Build history of the part. All positions in model axes, mm. A direction names the side the tool comes from. Coordinates: 2 decimals unless noted, no trailing zeros. Write each loop counter-clockwise with the first axis right and the second up, starting at its lowest first coordinate (ties: lowest second). Pieces come first, ordered by that corner, then holes.
```python
from build123d import *

# Parameters (mm, degrees)
SKETCH3_R   = 21.43125
SKETCH3_R_2 = 12.1539


with BuildPart() as part:
    # Sketch1 → Revolve1 (revolve)
    with BuildSketch(Plane.XY):
        Polygon((-11.786586159, -42.094950568), (8.688397797, -21.619966611), (5.298351111, -18.229919926), (-15.041929003, -38.839607724), align=None)
    revolve(axis=Axis((-26.940768363, -26.940768363, 0), (0.707106781, 0.707106781, 0)))



with BuildPart() as body_2:
    # Sketch2 → Revolve2 (revolve)
    with BuildSketch(Plane.XY):
        Polygon((16.8275, 38.1), (16.637, 9.144), (21.43125, 9.144), (21.43125, 38.1), align=None)
    revolve(axis=Axis((0, 0, 0), (0, 1, 0)))


with BuildPart() as part_1:
    add(part.part)

    add(body_2.part)  # Sweep1 merges body 2
    # Sweep1: sweep along a path in Sketch4
    with BuildLine(Plane.XY) as sweep1_path:
        ThreePointArc((-6.465784407, -6.465784407), (-1.680402618, 0.696045555), (0, 9.144))
    # Sketch3 → Sweep1 (sweep)
    with BuildSketch(Plane(origin=(-6.465784407, -6.465784407, 0), x_dir=(0, 0, -1), z_dir=(0.707106781, 0.707106781, 0))):
        Circle(SKETCH3_R)
        Circle(SKETCH3_R_2, mode=Mode.SUBTRACT)
    sweep(path=sweep1_path.line)


solid = part_1.part
```
1. Saw through at A-A on y = 31. List the corners of the cut face in (x, z), plus the area to 3 significant figures.
Computed values:
outline: circle Ø42.86 at (0, 0); hole circle Ø33.56 at (0, 0)
area: 558 mm2
2. Saw through at B-B on y = 4. State how many separate pieces and enclosed holes the cut face has, plus the area to 3 significant figures.
Computed values:
separate pieces: 1
enclosed holes: 2
area: 1,060 mm2
3. 3-axis set-ups, long thin cutter, end or side, ignore diameter. For faces 1 (the face through (11.52, 23.82, -18.07)), 2 (the face through (-7.28, -5.65, -12.25)), 3 (the face through (-13, 38.1, 11)): which of +Z, -Z, +X, -X, +Y, -Y reach the whole face in a straight line?
Computed values:
face 1: +Y
face 2: none
face 3: +Z, -Z, +X, -X, +Y
4. Flat gauge pins, fed straight in: pin 1 (2 mm diameter, centred on y = 23.5, z = -15, fed in from -X); pin 2 (1.5 mm diameter, centred on x = 2.5, y = 28.5, fed in from +Z); pin 3 (3 mm diameter, centred on x = -11.5, y = 4, fed in from -Z). Where does each tip first touch, or does it go through?
Computed values:
pin 1: stops at x = -16.23
pin 2: stops at z = 21.36
pin 3: stops at z = -19.53
5. Saw through at C-C on y = 12.5. List the corners of the cut face in (x, z).
Computed values:
outline: circle Ø42.86 at (0, 0); hole circle Ø33.32 at (0, 0)
6. Probe line 1 along X through (y, z) = (3.5, 3.5); line 2 along Z through (x, y) = (-5, -13); line 3 along Z through (x, y) = (-8, -3.5). List the from-to ranges inside material, lowest first.
Computed values:
line 1: x = -26.4 to -19.52, -16.43 to -13.3, 11.16 to 20.77
line 2: z = -20.67 to -15.67, 15.67 to 20.67
line 3: z = -21.2 to -11.74, 11.74 to 21.2
7. Mould opens along Y. For faces 4 (the face through (-33.605, -20.276, 14.187)), 5 (the face through (-7.5, 9.144, 9.8)), 6 (the face through (-18.39, -15.31, -16.59)) say: +Y half, -Y half, draft (parallel to the pull), parting line (faces both ways), or undercut.
Computed values:
face 4: -Y half
face 5: +Y half
face 6: undercut
